For this review, use the dimensioned drawing (mm, ordinates from the lowest corner) and the shaded views. Round coordinates to 2 decimals unless told otherwise and drop trailing zeros. Write each loop counter-clockwise with the first axis right and the second up, starting at its lowest first coordinate (ties: lowest second). Pieces come first, ordered by that corner, then holes. Notation, with made-up numbers: M 58,72 L 67,72 A11 ccw 67,90 Z; hole C 26.25,-32 d5. An arc over 180 degrees is marked long. One line per question, with ' | ' between items.
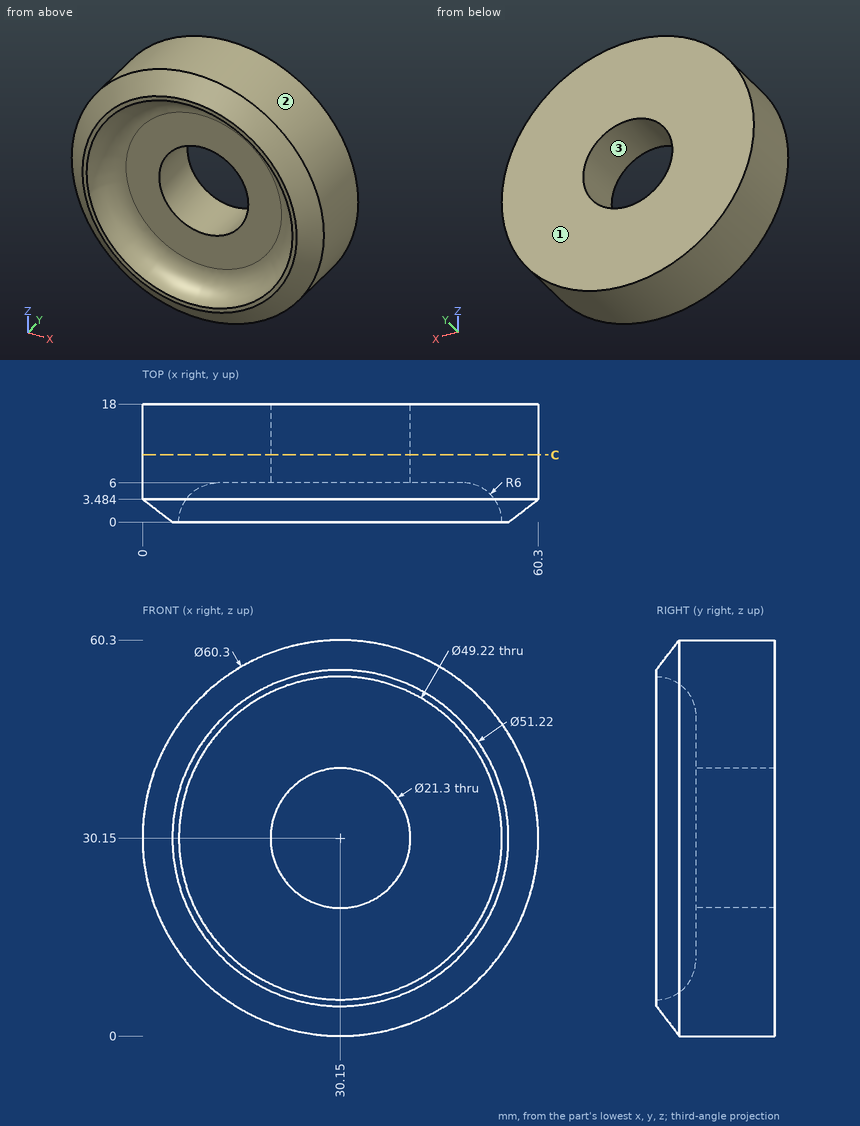
Item 1: Mouldability with a two-part tool opening along X and no side actions: class the marked faces 1, 2 and 3 as +X half, -X half, draft (parallel to the pull), parting line (faces both ways), or undercut.
Results:
face 1: draft | face 2: parting line | face 3: undercut
Item 2: Insertion check: pin 1 Ø1 at (x, y) = (13, 15) entering from -Z (1 decimal); pin 2 Ø5 at (y, z) = (7.5, 52) entering from +X; pin 3 Ø8 at (y, z) = (4, 50.5) entering from +X. Each pin has a flat end and moves straight along its axis. Give the tip position at first contact, or say it passes through.
Results:
pin 1: z = 5 | pin 2: x = 53.27 | pin 3: x = 55.48
Item 3: To check wall thickness, follow line 1 along Z through (x, y) = (30.15, 10.5); line 2 along Y through (x, z) = (35, 12); line 3 along Z through (x, y) = (32.5, 11). State the ranges of each line that lie inside material, in increasing order. Write a range as from..to.
Results:
line 1: 0..19.5, 40.8..60.3 | line 2: 6..18 | line 3: 0.09..19.76, 40.54..60.21
Item 4: Take a section at C-C (y = 10.25). Write out the cut boundary in (x, z), then the cut area to 3 significant figures.
Results:
outline: C 30.15,30.15 d60.3; hole C 30.15,30.15 d21.3 | area: 2,500 mm2
